```python
from build123d import *

# Parameters (mm, degrees)
BOSS_EXTRUDE1_DEPTH     = 5
CUT_EXTRUDE1_DEPTH      = 81.777472107
SKETCH3_R               = 3
BOSS_EXTRUDE2_DEPTH     = 7
CUT_EXTRUDE2_DEPTH      = 82.510735489
CUT_EXTRUDE2_DEPTH_BACK = 82.510735489
SKETCH4_R               = 2.05
SKETCH5_W               = 12
SKETCH5_H               = 56
CUT_EXTRUDE3_DEPTH      = 81.925892025
FILLET1_R               = 3
SKETCH6_W               = 50
SKETCH6_H               = 4
CUT_EXTRUDE4_DEPTH      = 81.925892025
SKETCH7_W               = 7.2
SKETCH7_H               = 8
BOSS_EXTRUDE3_DEPTH     = 3
SKETCH8_R               = 2.05
CUT_EXTRUDE5_DEPTH      = 6
MIRROR4_COPY_1_SKETCH_W = 7.2
MIRROR4_COPY_1_SKETCH_H = 8
MIRROR4_COPY_1_DEPTH    = 3
MIRROR4_COPY_2_SKETCH_R = 2.05
MIRROR4_COPY_2_DEPTH    = 6
SKETCH10_W              = 111.8
SKETCH10_H              = 1
CUT_EXTRUDE7_DEPTH      = 81.925892025
FILLET5_R               = 2
SKETCH11_W              = 8
SKETCH11_H              = 56
BOSS_EXTRUDE4_DEPTH     = 5
SKETCH12_W              = 18
SKETCH12_H              = 40
CUT_EXTRUDE8_DEPTH      = 81.436310209
FILLET6_R               = 3
CUT_EXTRUDE9_DEPTH      = 81.436310209
CUT_EXTRUDE9_DEPTH_BACK = 81.436310209
SKETCH13_W              = 111.8
SKETCH13_H              = 2.1
SKETCH13_H_2            = 1.9
SKETCH14_W              = 6.5
SKETCH14_H              = 7
BOSS_EXTRUDE5_DEPTH     = 6
SKETCH15_R              = 1.65
CUT_EXTRUDE10_DEPTH     = 6
CUT_EXTRUDE11_START     = -6
SKETCH16_R              = 1.65
CUT_EXTRUDE11_DEPTH     = 6


# Some blends are built 0.0001 mm under size
with BuildPart() as part:
    # Sketch1 → Boss-Extrude1 (new body)
    with BuildSketch(Plane(origin=(0, 0, 0), x_dir=(1, 0, 0), z_dir=(0, 1, 0))):
        Polygon((-70, -32.9), (-70, 32.9), (-55.9, 32.9), (-55.9, 40), (55.9, 40), (55.9, 32.9), (70, 32.9), (70, -32.9), (55.9, -32.9), (55.9, -40), (-55.9, -40), (-55.9, -32.9), align=None)
    extrude(amount=BOSS_EXTRUDE1_DEPTH)

    # Sketch2 → Cut-Extrude1 (cut, through all)
    with BuildSketch(Plane(origin=(0, 5, 0), x_dir=(1, 0, 0), z_dir=(0, 1, 0))):
        Polygon((-41, 26), (-38, 26), (-38, 29), (38, 29), (38, 26), (41, 26), (41, -30), (38, -30), (38, -33), (-38, -33), (-38, -30), (-41, -30), align=None)
    extrude(amount=-CUT_EXTRUDE1_DEPTH, mode=Mode.SUBTRACT)

    # Sketch3 → Boss-Extrude2 (add)
    with BuildSketch(Plane(origin=(0, 5, 0), x_dir=(1, 0, 0), z_dir=(0, 1, 0))):
        with Locations(Location((-41, -33, 0), (0, 0, 90))):
            Circle(SKETCH3_R)
        with Locations(Location((41, -33, 0), (0, 0, 90))):
            Circle(SKETCH3_R)
        with Locations(Location((41, 29, 0), (0, 0, 270))):
            Circle(SKETCH3_R)
        with Locations(Location((-41, 29, 0), (0, 0, 270))):
            Circle(SKETCH3_R)
    extrude(amount=BOSS_EXTRUDE2_DEPTH)

    # Sketch4 → Cut-Extrude2 (cut, two sides: drawn at the far end of the back side and taken through both)
    with BuildSketch(Plane(origin=(0, 12, 0), x_dir=(1, 0, 0), z_dir=(0, 1, 0)).offset(-CUT_EXTRUDE2_DEPTH_BACK)):
        with Locations(Location((-41, 29, 0), (0, 0, 270))):
            Circle(SKETCH4_R)
        with Locations(Location((41, 29, 0), (0, 0, 270))):
            Circle(SKETCH4_R)
        with Locations(Location((41, -33, 0), (0, 0, 270))):
            Circle(SKETCH4_R)
        with Locations(Location((-41, -33, 0), (0, 0, 270))):
            Circle(SKETCH4_R)
    extrude(amount=CUT_EXTRUDE2_DEPTH + CUT_EXTRUDE2_DEPTH_BACK, mode=Mode.SUBTRACT)

    # Sketch5 → Cut-Extrude3 (cut, through all)
    with BuildSketch(Plane(origin=(0, 5, 0), x_dir=(1, 0, 0), z_dir=(0, 1, 0))):
        with Locations((-47, -2)):
            Rectangle(SKETCH5_W, SKETCH5_H)
        with Locations((47, -2)):
            Rectangle(SKETCH5_W, SKETCH5_H)
    extrude(amount=-CUT_EXTRUDE3_DEPTH, mode=Mode.SUBTRACT)

    # Fillet1
    fillet1_edges = [part.edges().sort_by_distance(p)[0] for p in [
        (38, 2.5, 30),
        (-38, 2.5, 30),
        (38, 2.5, -26),
        (-38, 2.5, -26),
    ]]
    fillet(fillet1_edges, radius=FILLET1_R - 0.0001)  # a hair under: the kernel refuses the full size

    # Sketch6 → Cut-Extrude4 (cut, through all)
    with BuildSketch(Plane(origin=(0, 5, 0), x_dir=(1, 0, 0), z_dir=(0, 1, 0))):
        with Locations((0, 31)):
            Rectangle(SKETCH6_W, SKETCH6_H)
    extrude(amount=-CUT_EXTRUDE4_DEPTH, mode=Mode.SUBTRACT)

    # Sketch7 → Boss-Extrude3 (add)
    with BuildSketch(Plane(origin=(0, 5, 0), x_dir=(1, 0, 0), z_dir=(0, 1, 0))):
        with Locations((59.5, 28.9)):
            Rectangle(SKETCH7_W, SKETCH7_H)
    boss_extrude3 = extrude(amount=BOSS_EXTRUDE3_DEPTH)

    # Sketch8 → Cut-Extrude5 (cut)
    with BuildSketch(Plane(origin=(0, 0, -32.9), x_dir=(-1, 0, 0), z_dir=(0, 0, -1))):
        with Locations((-59.5, 4)):
            Circle(SKETCH8_R)
    cut_extrude5 = extrude(amount=-CUT_EXTRUDE5_DEPTH, mode=Mode.SUBTRACT)

    # Mirror3: Boss-Extrude3, Cut-Extrude5 across plane
    add(boss_extrude3.mirror(Plane(origin=(0, 0, 0), x_dir=(0, 0, 1), z_dir=(1, 0, 0))))
    add(cut_extrude5.mirror(Plane(origin=(0, 0, 0), x_dir=(0, 0, 1), z_dir=(1, 0, 0))), mode=Mode.SUBTRACT)

    # Mirror4: Boss-Extrude3, Cut-Extrude5 across plane
    add(boss_extrude3.mirror(Plane.XY))
    add(cut_extrude5.mirror(Plane.XY), mode=Mode.SUBTRACT)

    # Mirror4 copy 1 sketch → Mirror4 copy 1 (add)
    with BuildSketch(Plane(origin=(0, 5, 0), x_dir=(-1, 0, 0), z_dir=(0, 1, 0))):
        with Locations((59.5, 28.9)):
            Rectangle(MIRROR4_COPY_1_SKETCH_W, MIRROR4_COPY_1_SKETCH_H)
    extrude(amount=MIRROR4_COPY_1_DEPTH)

    # Mirror4 copy 2 sketch → Mirror4 copy 2 (cut)
    with BuildSketch(Plane.XY.offset(32.9)):
        with Locations((-59.5, 4)):
            Circle(MIRROR4_COPY_2_SKETCH_R)
    extrude(amount=-MIRROR4_COPY_2_DEPTH, mode=Mode.SUBTRACT)

    # Sketch10 → Cut-Extrude7 (cut, through all)
    with BuildSketch(Plane(origin=(0, 5, 0), x_dir=(1, 0, 0), z_dir=(0, 1, 0))):
        with Locations((0, 39.5)):
            Rectangle(SKETCH10_W, SKETCH10_H)
        with Locations((0, -39.5)):
            Rectangle(SKETCH10_W, SKETCH10_H)
    extrude(amount=-CUT_EXTRUDE7_DEPTH, mode=Mode.SUBTRACT)

    # Fillet5
    # the kernel refuses this fillet: 2 mm, written as the material it adds along each edge
    with BuildSketch(Plane(origin=(41, 5, 33), x_dir=(-1, 0, 0), z_dir=(0, 0, -1))) as fillet5_piece_1_section:
        with BuildLine():
            CenterArc((3 + FILLET5_R, FILLET5_R), FILLET5_R, 180, 90)
            Line((3, FILLET5_R), (3, 0))
            Line((3, 0), (3 + FILLET5_R, 0))
        make_face()
    fillet5_piece_1 = revolve(axis=Axis((41, 5, 33), (0, 1, 0)), revolution_arc=270, mode=Mode.PRIVATE)
    fillet5_piece_1 = split(fillet5_piece_1, bisect_by=Plane(origin=(37.573130255, 5.322558535, 30), z_dir=(0, 0, 1)), keep=Keep.TOP, mode=Mode.PRIVATE)
    add(fillet5_piece_1)
    with BuildSketch(Plane(origin=(-41, 5, 33), x_dir=(0, 0, -1), z_dir=(1, 0, 0))) as fillet5_piece_2_section:
        with BuildLine():
            CenterArc((3 + FILLET5_R, FILLET5_R), FILLET5_R, 180, 90)
            Line((3, FILLET5_R), (3, 0))
            Line((3, 0), (3 + FILLET5_R, 0))
        make_face()
    fillet5_piece_2 = revolve(axis=Axis((-41, 5, 33), (0, 1, 0)), revolution_arc=270, mode=Mode.PRIVATE)
    fillet5_piece_2 = split(fillet5_piece_2, bisect_by=Plane(origin=(-43.742596375, 5.466410384, 30), z_dir=(0, 0, 1)), keep=Keep.TOP, mode=Mode.PRIVATE)
    add(fillet5_piece_2)
    with BuildSketch(Plane(origin=(41, 5, -29), x_dir=(0, 0, 1), z_dir=(-1, 0, 0))) as fillet5_piece_3_section:
        with BuildLine():
            CenterArc((3 + FILLET5_R, FILLET5_R), FILLET5_R, 180, 90)
            Line((3, FILLET5_R), (3, 0))
            Line((3, 0), (3 + FILLET5_R, 0))
        make_face()
    fillet5_piece_3 = revolve(axis=Axis((41, 5, -29), (0, 1, 0)), revolution_arc=270, mode=Mode.PRIVATE)
    fillet5_piece_3 = split(fillet5_piece_3, bisect_by=Plane(origin=(43.742596375, 5.466410384, -26), z_dir=(0, 0, -1)), keep=Keep.TOP, mode=Mode.PRIVATE)
    add(fillet5_piece_3)
    with BuildSketch(Plane(origin=(-41, 5, -29), x_dir=(1, 0, 0), z_dir=(0, 0, 1))) as fillet5_piece_4_section:
        with BuildLine():
            CenterArc((3 + FILLET5_R, FILLET5_R), FILLET5_R, 180, 90)
            Line((3 + FILLET5_R, 0), (3, 0))
            Line((3, 0), (3, FILLET5_R))
        make_face()
    fillet5_piece_4 = revolve(axis=Axis((-41, 5, -29), (0, 1, 0)), revolution_arc=270, mode=Mode.PRIVATE)
    fillet5_piece_4 = split(fillet5_piece_4, bisect_by=Plane(origin=(-41, 5.571713042, -26), z_dir=(0, 0, -1)), keep=Keep.TOP, mode=Mode.PRIVATE)
    add(fillet5_piece_4)

    # Sketch11 → Boss-Extrude4 (add)
    with BuildSketch(Plane(origin=(0, 5, 0), x_dir=(1, 0, 0), z_dir=(0, 1, 0))):
        with Locations((49, -2)):
            Rectangle(SKETCH11_W, SKETCH11_H)
        with Locations((-49, -2)):
            Rectangle(SKETCH11_W, SKETCH11_H)
    extrude(amount=-BOSS_EXTRUDE4_DEPTH)

    # Sketch12 → Cut-Extrude8 (cut, symmetric)
    with BuildSketch(Plane(origin=(0, 5, 0), x_dir=(1, 0, 0), z_dir=(0, 1, 0))):
        with Locations((54, 0)):
            Rectangle(SKETCH12_W, SKETCH12_H)
    cut_extrude8 = extrude(amount=CUT_EXTRUDE8_DEPTH, both=True, mode=Mode.SUBTRACT)

    # Mirror7: Cut-Extrude8 across plane
    add(cut_extrude8.mirror(Plane(origin=(0, 0, 0), x_dir=(0, 0, 1), z_dir=(1, 0, 0))), mode=Mode.SUBTRACT)

    # Fillet6
    fillet6_edges = [part.edges().sort_by_distance(p)[0] for p in [
        (45, 2.5, 20),
        (45, 2.5, -20),
        (-45, 2.5, -20),
        (-45, 2.5, 20),
    ]]
    fillet(fillet6_edges, radius=FILLET6_R)

    # Sketch13 → Cut-Extrude9 (cut, two sides: drawn at the far end of the back side and taken through both)
    with BuildSketch(Plane(origin=(0, 5, 0), x_dir=(1, 0, 0), z_dir=(0, 1, 0)).offset(-CUT_EXTRUDE9_DEPTH_BACK)):
        with Locations((0, 37.95)):
            Rectangle(SKETCH13_W, SKETCH13_H)
        with Locations((0, -38.05)):
            Rectangle(SKETCH13_W, SKETCH13_H_2)
    extrude(amount=CUT_EXTRUDE9_DEPTH + CUT_EXTRUDE9_DEPTH_BACK, mode=Mode.SUBTRACT)

    # Sketch14 → Boss-Extrude5 (add)
    with BuildSketch(Plane(origin=(0, 5, 0), x_dir=(1, 0, 0), z_dir=(0, 1, 0))):
        with Locations((-52.65, -33.6)):
            Rectangle(SKETCH14_W, SKETCH14_H)
        with Locations((-52.65, 33.4)):
            Rectangle(SKETCH14_W, SKETCH14_H)
    boss_extrude5 = extrude(amount=BOSS_EXTRUDE5_DEPTH)

    # Sketch15 → Cut-Extrude10 (cut)
    with BuildSketch(Plane.XY.offset(37.1)):
        with Locations((-52.9, 2.5)):
            Circle(SKETCH15_R)
        with Locations((-52.9, 8.5)):
            Circle(SKETCH15_R)
    cut_extrude10 = extrude(amount=-CUT_EXTRUDE10_DEPTH, mode=Mode.SUBTRACT)

    # Sketch16 → Cut-Extrude11 (cut)
    with BuildSketch(Plane(origin=(0, 0, -36.9), x_dir=(-1, 0, 0), z_dir=(0, 0, -1)).offset(CUT_EXTRUDE11_START)):
        with Locations(Location((52.9, 8.5, 0), (0, 0, 180))):
            Circle(SKETCH16_R)
        with Locations(Location((52.9, 2.5, 0), (0, 0, 180))):
            Circle(SKETCH16_R)
    cut_extrude11 = extrude(amount=CUT_EXTRUDE11_DEPTH, mode=Mode.SUBTRACT)

    # Mirror8: Boss-Extrude5, Cut-Extrude10, Cut-Extrude11 across plane
    add(boss_extrude5.mirror(Plane(origin=(0, 0, 0), x_dir=(0, 0, 1), z_dir=(1, 0, 0))))
    add(cut_extrude10.mirror(Plane(origin=(0, 0, 0), x_dir=(0, 0, 1), z_dir=(1, 0, 0))), mode=Mode.SUBTRACT)
    add(cut_extrude11.mirror(Plane(origin=(0, 0, 0), x_dir=(0, 0, 1), z_dir=(1, 0, 0))), mode=Mode.SUBTRACT)


solid = part.part
```
Build history of the part. All positions in model axes, mm. A direction names the side the tool comes from. Round coordinates to 2 decimals unless told otherwise and drop trailing zeros. Write each loop counter-clockwise with the first axis right and the second up, starting at its lowest first coordinate (ties: lowest second). Pieces come first, ordered by that corner, then holes.
1) Drill centre lines: probe 1 along X at (y, z) = (2.5, -6); probe 2 along Z at (x, y) = (-11.5, 0.75); probe 3 along Y at (x, z) = (52, 34). Where is each one in solid material? Low to high.
2) Pin check, flat tips, straight feed: pin 1 (3 mm diameter, centred on x = 52.9, y = 8.5, fed in from +Z); pin 2 (2 mm diameter, centred on x = 53, z = 33.5, fed in from +Y); pin 3 (3.5 mm diameter, centred on x = -41, z = 33, fed in from -Y); pin 4 (2 mm diameter, centred on y = 5.5, z = 35, fed in from +X). Stop position of each tip, or through.
3) Band-saw the part on A-A, the plane x = -3.5. List the corners of the cut face in (y, z).
4) Band-saw the part on C-C, the plane x = -52.9. List the corners of the cut face in (y, z).
5) Mould opens along X. For faces 1 (the flat face through (63, 3, -32.9)), 2 (the cylindrical face through (38.9, 2.46, 30.86)), 3 (the flat face through (-63.1, 6, 29)) say: +X half, -X half, draft (parallel to the pull), parting line (faces both ways), or undercut.
6) Band-saw the part on B-B, the plane z = 7. List the corners of the cut face in (x, y).
7) 3-axis set-ups, long thin cutter, end or side, ignore diameter. For faces 4 (the flat face through (-53, 3, 31.1)), 5 (the flat face through (-55.9, 6, -27)), 6 (the flat face through (55, 3, -20)): which of +Z, -Z, +X, -X, +Y, -Y reach the whole face in a straight line?
Ans:
1. probe 1: x = -70 to -63, 63 to 70
1. probe 2: z = -36.9 to -33, 33 to 37.1
1. probe 3: y = 0 to 1.12, 3.88 to 7.12, 9.88 to 11
2. pin 1: stops at z = 31.1
2. pin 2: stops at y = 11
2. pin 3: passes through
2. pin 4: stops at x = 55.9
3. outline: (0, -36.9) - (5, -36.9) - (5, -33) - (0, -33) - close; (0, 33) - (5, 33) - (5, 37.1) - (0, 37.1) - close
4. outline: (0, -36.9) - (0.85, -36.9) - (0.85, -30.9) - (4.15, -30.9) - (4.15, -36.9) - (6.85, -36.9) - (6.85, -30.9) - (10.15, -30.9) - (10.15, -36.9) - (11, -36.9) - (11, -29.9) - (5, -29.9) - (5, -20) - (0, -20) - close; (0, 20) - (5, 20) - (5, 30.1) - (11, 30.1) - (11, 37.1) - (10.15, 37.1) - (10.15, 31.1) - (6.85, 31.1) - (6.85, 37.1) - (4.15, 37.1) - (4.15, 31.1) - (0.85, 31.1) - (0.85, 37.1) - (0, 37.1) - close
5. face 1: draft
5. face 2: undercut
5. face 3: -X half
6. outline: (-70, 0) - (-63, 0) - (-63, 5) - (-70, 5) - close; (63, 0) - (70, 0) - (70, 5) - (63, 5) - close
7. face 4: +Z
7. face 5: +Y
7. face 6: +Y, -Y
